Read the model definition and answer for the solid it produces. Units are mm, in the model's axes. A direction names the side the tool comes from. Coordinates: 2 decimals unless noted, no trailing zeros. Write each loop counter-clockwise with the first axis right and the second up, starting at its lowest first coordinate (ties: lowest second). Pieces come first, ordered by that corner, then holes. Notation, with made-up numbers: (78.5, 55) -> (90.5, 55) arc R23 cw to (90.5, 77) -> close; hole circle Ø9 at (-9, 16). An arc over 180 degrees is marked (long way). Return JSON: item names as keys, results as strings.
from build123d import *
from build123d import SkipClean  # not in build123d's __all__

# Parameters (mm, degrees)
F0_W      = 101.6
F0_H      = 76.2
F1_DEPTH  = 50.8
F2_R      = 12.7
F4_DEPTH  = 25.4
F9_R      = 7.3504137181
F10_DEPTH = 25.4


# Not quite as in the source:
# - after a boolean that leaves OpenCascade's solid faulty, fix() repairs it
# - the program builds the solid bodies; features that only make, move or delete a surface that nothing else refers to are left out


with BuildPart() as f1:
    # F0 (on Top) → F1 (new body)
    with BuildSketch(Plane.XY):
        with Locations((50.8, 38.1)):
            Rectangle(F0_W, F0_H)
    extrude(amount=F1_DEPTH)

    # F2
    f2_edges = [f1.edges().sort_by_distance(p)[0] for p in [
        (0, 0, 25.4),
        (101.6, 0, 25.4),
        (101.6, 76.2, 25.4),
        (0, 76.2, 25.4),
    ]]
    fillet(f2_edges, radius=F2_R)

    # F3 (on face) → F4 (join)
    with BuildSketch(Plane.XY.offset(50.8)):
        with BuildLine():
            ThreePointArc((0, 63.5), (3.7197438789, 54.5197438789), (12.7, 50.8))
            Line((12.7, 50.8), (25.4, 50.8))
            Line((25.4, 50.8), (25.4, 63.5))
            ThreePointArc((25.4, 63.5), (21.6802561211, 72.4802561211), (12.7, 76.2))
            ThreePointArc((12.7, 76.2), (3.7197438789, 72.4802561211), (0, 63.5))
        make_face()
    with SkipClean():  # cleaning this boolean's faces spoils the solid; the shape is the same uncleaned
        extrude(amount=F4_DEPTH)

    # F9 (on face) → F10 (cut)
    with BuildSketch(Plane.XY.offset(50.8)):
        with Locations((85.2179154754, 58.332465589)):
            Circle(F9_R)
    extrude(amount=-F10_DEPTH, mode=Mode.SUBTRACT)

    add(f1.part.fix(), mode=Mode.REPLACE)


solid = f1.part
1. Flat-ended cylindrical pins translate along their axes: pin 1 Ø14 at (x, z) = (18.5, 60) entering from -Y; pin 2 Ø16 at (x, y) = (88, 60) entering from +Z; pin 3 Ø6.5 at (y, z) = (60, 60.5) entering from +X. Find the tip coordinate at first contact, or state that the pin passes through.
Taken from the geometry:
{"pin 1": "stops at y = 50.8", "pin 2": "stops at z = 50.8", "pin 3": "stops at x = 25.4"}
2. A tool of negligible diameter and unlimited length cuts with its end or side. For faces 5 (the face through (25.4, 57, 63)), 6 (the face through (19, 50.8, 63)), 7 (the face through (13, 64, 76.2)), from which of +Z, -Z, +X, -X, +Y, -Y can it reach the whole face along a straight path? Write none if from no direction.
Taken from the geometry:
{"face 5": "+Z, +X, +Y, -Y", "face 6": "+Z, +X, -X, -Y", "face 7": "+Z, +X, -X, +Y, -Y"}
3. The part is cut by section D-D (x = 79.5). Determine the outline of the cut face in (y, z).
Taken from the geometry:
{"outline": "(0, 0) -> (76.2, 0) -> (76.2, 50.8) -> (62.95, 50.8) -> (62.95, 25.4) -> (53.71, 25.4) -> (53.71, 50.8) -> (0, 50.8) -> close"}
4. The part is cut by section B-B (z = 42.5). Determine the outline of the cut face in (x, y), then the cut area to 3 significant figures.
Taken from the geometry:
{"outline": "(0, 12.7) arc R12.7 ccw to (12.7, 0) -> (88.9, 0) arc R12.7 ccw to (101.6, 12.7) -> (101.6, 63.5) arc R12.7 ccw to (88.9, 76.2) -> (12.7, 76.2) arc R12.7 ccw to (0, 63.5) -> close; hole circle Ø14.7 at (85.22, 58.33)", "area": "7,430 mm2"}
5. For a pull along X with two mould halves and no side action, classify faces 1 (the face through (92.23, 60.54, 38.28)), 2 (the face through (97.78, 3.62, 25.76)), 3 (the face through (85, 58, 25.4)), 4 (the face through (0, 38, 25)) as +X half, -X half, draft (parallel to the pull), parting line (faces both ways), or undercut.
Taken from the geometry:
{"face 1": "undercut", "face 2": "+X half", "face 3": "undercut", "face 4": "-X half"}
6. Consider L1, parallel to Z at x = 29, y = 63; L2, parallel to Y at x = 90, z = 39.5; L3, parallel to X at y = 11.5, z = 44.5. Determine where each line is inside the solid, lowest interval first.
Taken from the geometry:
{"L1": "z = 0 to 50.8", "L2": "y = 0.05 to 52.75, 63.91 to 76.15", "L3": "x = 0.06 to 101.54"}
7. The part is cut by section A-A (z = 7). Determine the outline of the cut face in (x, y), then the cut area to 3 significant figures.
Taken from the geometry:
{"outline": "(0, 12.7) arc R12.7 ccw to (12.7, 0) -> (88.9, 0) arc R12.7 ccw to (101.6, 12.7) -> (101.6, 63.5) arc R12.7 ccw to (88.9, 76.2) -> (12.7, 76.2) arc R12.7 ccw to (0, 63.5) -> close", "area": "7,600 mm2"}
8. The part is cut by section C-C (y = 54). Determine the outline of the cut face in (x, z), then the cut area to 3 significant figures.
Taken from the geometry:
{"outline": "(0, 0) -> (101.6, 0) -> (101.6, 50.8) -> (91.16, 50.8) -> (91.16, 25.4) -> (79.28, 25.4) -> (79.28, 50.8) -> (25.4, 50.8) -> (25.4, 76.2) -> (4.27, 76.2) -> (4.27, 50.8) -> (0, 50.8) -> close", "area": "5,400 mm2"}
